```python
from build123d import *

# Parameters (mm, degrees)
BASE_DEPTH          = 3
SERVO_SUPPORT_DEPTH = 43.8
SKETCH21_W          = 6
SKETCH21_H          = 4.65
SERVO_MOUNTS_DEPTH  = 12.4
SERVO_SCREWS_REACH  = 142.173
SKETCH22_R          = 1.3
FILLET1_R           = 2
SKETCH23_W          = 16.5
SKETCH23_H          = 31.3
SHAFT_SUPPORT_DEPTH = 3
SKETCH24_W          = 5.5
SKETCH24_H          = 31.3
BOSS_EXTRUDE6_DEPTH = 56.2
FILLET2_R           = 8
FILLET3_R           = 8
SHAFT_REACH         = 151.771
SKETCH25_R          = 1.7
SCREWS_REACH        = 107.316
SKETCH26_R          = 1.6
SKETCH26_R_2        = 1.4
SKETCH31_W          = 7
SKETCH31_H          = 13.5765
BOSS_EXTRUDE8_DEPTH = 5
SKETCH30_R          = 2.5
BOSS_EXTRUDE9_DEPTH = 2.5
CUT_EXTRUDE1_REACH  = 122.29
SKETCH32_R          = 1.15
CHAMFER1_SIZE       = 2.5
CHAMFER2_SIZE       = 4


with BuildPart() as part:
    # Sketch19 → Base (new body)
    with BuildSketch(Plane.XY):
        Polygon((61.5, 19.3), (56.5, 19.3), (34, 29.3), (34, 34.3), (-59.5, 34.3), (-59.5, -43), (61.5, -43), align=None)
    extrude(amount=BASE_DEPTH)

    # Sketch20 → Servo support (add)
    with BuildSketch(Plane.XY):
        Polygon((-53.298152188, -10.85), (-55.448152188, -10.85), (-59.5, -10.85), (-59.5, 21.25), (-55.448152188, 21.25), (-53.298152188, 21.25), (-45.748152188, 21.25), (-45.748152188, 8.609473612), (-45.748152188, -10.85), align=None)
    extrude(amount=SERVO_SUPPORT_DEPTH)

    # Sketch21 → Servo mounts (add)
    with BuildSketch(Plane.XY.offset(43.8)):
        with Locations((-56.5, -8.525)):
            Rectangle(SKETCH21_W, SKETCH21_H)
        with Locations((-56.5, 18.925)):
            Rectangle(SKETCH21_W, SKETCH21_H)
    extrude(amount=SERVO_MOUNTS_DEPTH)

    # Sketch22 → Servo screws (cut, up to next)
    with BuildSketch(Plane.ZY.offset(59.5), mode=Mode.PRIVATE) as servo_screws_sk1:
        with Locations(Location((50, -8.65, 0), (0, 0, 270))):
            Circle(SKETCH22_R)
    servo_screws_tool1 = extrude(servo_screws_sk1.sketch, amount=-SERVO_SCREWS_REACH, mode=Mode.PRIVATE) & part.part
    # Sketch22 → Servo screws (cut, up to next)
    with BuildSketch(Plane.ZY.offset(59.5), mode=Mode.PRIVATE) as servo_screws_sk2:
        with Locations(Location((50, 19.05, 0), (0, 0, 270))):
            Circle(SKETCH22_R)
    servo_screws_tool2 = extrude(servo_screws_sk2.sketch, amount=-SERVO_SCREWS_REACH, mode=Mode.PRIVATE) & part.part
    add(servo_screws_tool1.solids().sort_by_distance((-59.5, -8.65, 50))[0], mode=Mode.SUBTRACT)
    add(servo_screws_tool2.solids().sort_by_distance((-59.5, 19.05, 50))[0], mode=Mode.SUBTRACT)

    # Fillet1
    fillet1_edges = [part.edges().sort_by_distance(p)[0] for p in [
        (-56.5, 21.25, 56.2),
        (-56.5, -10.85, 56.2),
    ]]
    fillet(fillet1_edges, radius=FILLET1_R)

    # Sketch23 → Shaft support (add)
    with BuildSketch(Plane.XY):
        with Locations((69.75, 3.65)):
            Rectangle(SKETCH23_W, SKETCH23_H)
    extrude(amount=SHAFT_SUPPORT_DEPTH)

    # Sketch24 → Boss-Extrude6 (add)
    with BuildSketch(Plane.XY):
        with Locations((75.25, 3.65)):
            Rectangle(SKETCH24_W, SKETCH24_H)
    extrude(amount=BOSS_EXTRUDE6_DEPTH)

    # Fillet2
    fillet2_edges = [part.edges().sort_by_distance(p)[0] for p in [
        (61.5, -12, 1.5),
    ]]
    fillet(fillet2_edges, radius=FILLET2_R)

    # Fillet3
    fillet3_edges = [part.edges().sort_by_distance(p)[0] for p in [
        (75.25, 19.3, 56.2),
        (75.25, -12, 56.2),
    ]]
    fillet(fillet3_edges, radius=FILLET3_R)

    # Sketch25 → Shaft (cut, up to next)
    with BuildSketch(Plane.ZY.offset(-72.5), mode=Mode.PRIVATE) as shaft_sk1:
        with Locations((50, 0)):
            Circle(SKETCH25_R)
    shaft_tool1 = extrude(shaft_sk1.sketch, amount=-SHAFT_REACH, mode=Mode.PRIVATE) & part.part
    add(shaft_tool1.solids().sort_by_distance((72.5, 0, 50))[0], mode=Mode.SUBTRACT)

    # Sketch26 → Screws (cut, up to next)
    with BuildSketch(Plane.XY, mode=Mode.PRIVATE) as screws_sk1:
        with Locations((-57, -40.5)):
            Circle(SKETCH26_R)
    screws_tool1 = extrude(screws_sk1.sketch, amount=SCREWS_REACH, mode=Mode.PRIVATE) & part.part
    # Sketch26 → Screws (cut, up to next)
    with BuildSketch(Plane.XY, mode=Mode.PRIVATE) as screws_sk2:
        with Locations((-10, -40.5)):
            Circle(SKETCH26_R)
    screws_tool2 = extrude(screws_sk2.sketch, amount=SCREWS_REACH, mode=Mode.PRIVATE) & part.part
    # Sketch26 → Screws (cut, up to next)
    with BuildSketch(Plane.XY, mode=Mode.PRIVATE) as screws_sk3:
        with Locations((59, -32)):
            Circle(SKETCH26_R)
    screws_tool3 = extrude(screws_sk3.sketch, amount=SCREWS_REACH, mode=Mode.PRIVATE) & part.part
    # Sketch26 → Screws (cut, up to next)
    with BuildSketch(Plane.XY, mode=Mode.PRIVATE) as screws_sk4:
        with Locations((59, 16.8)):
            Circle(SKETCH26_R)
    screws_tool4 = extrude(screws_sk4.sketch, amount=SCREWS_REACH, mode=Mode.PRIVATE) & part.part
    # Sketch26 → Screws (cut, up to next)
    with BuildSketch(Plane.XY, mode=Mode.PRIVATE) as screws_sk5:
        with Locations((31.5, 31.8)):
            Circle(SKETCH26_R)
    screws_tool5 = extrude(screws_sk5.sketch, amount=SCREWS_REACH, mode=Mode.PRIVATE) & part.part
    # Sketch26 → Screws (cut, up to next)
    with BuildSketch(Plane.XY, mode=Mode.PRIVATE) as screws_sk6:
        with Locations((-32.5, 31.8)):
            Circle(SKETCH26_R)
    screws_tool6 = extrude(screws_sk6.sketch, amount=SCREWS_REACH, mode=Mode.PRIVATE) & part.part
    # Sketch26 → Screws (cut, up to next)
    with BuildSketch(Plane.XY, mode=Mode.PRIVATE) as screws_sk7:
        with Locations((-57, 25.3)):
            Circle(SKETCH26_R)
    screws_tool7 = extrude(screws_sk7.sketch, amount=SCREWS_REACH, mode=Mode.PRIVATE) & part.part
    # Sketch26 → Screws (cut, up to next)
    with BuildSketch(Plane.XY, mode=Mode.PRIVATE) as screws_sk8:
        with Locations((-57, -14.5)):
            Circle(SKETCH26_R_2)
    screws_tool8 = extrude(screws_sk8.sketch, amount=SCREWS_REACH, mode=Mode.PRIVATE) & part.part
    # Sketch26 → Screws (cut, up to next)
    with BuildSketch(Plane.XY, mode=Mode.PRIVATE) as screws_sk9:
        with Locations((45.5, -40.5)):
            Circle(SKETCH26_R_2)
    screws_tool9 = extrude(screws_sk9.sketch, amount=SCREWS_REACH, mode=Mode.PRIVATE) & part.part
    add(screws_tool1.solids().sort_by_distance((-57, -40.5, 0))[0], mode=Mode.SUBTRACT)
    add(screws_tool2.solids().sort_by_distance((-10, -40.5, 0))[0], mode=Mode.SUBTRACT)
    add(screws_tool3.solids().sort_by_distance((59, -32, 0))[0], mode=Mode.SUBTRACT)
    add(screws_tool4.solids().sort_by_distance((59, 16.8, 0))[0], mode=Mode.SUBTRACT)
    add(screws_tool5.solids().sort_by_distance((31.5, 31.8, 0))[0], mode=Mode.SUBTRACT)
    add(screws_tool6.solids().sort_by_distance((-32.5, 31.8, 0))[0], mode=Mode.SUBTRACT)
    add(screws_tool7.solids().sort_by_distance((-57, 25.3, 0))[0], mode=Mode.SUBTRACT)
    add(screws_tool8.solids().sort_by_distance((-57, -14.5, 0))[0], mode=Mode.SUBTRACT)
    add(screws_tool9.solids().sort_by_distance((45.5, -40.5, 0))[0], mode=Mode.SUBTRACT)

    # Sketch31 → Boss-Extrude8 (add)
    with BuildSketch(Plane.XZ.offset(43)):
        with Locations((0, 9.78825)):
            Rectangle(SKETCH31_W, SKETCH31_H)
        with Locations((58, 9.78825)):
            Rectangle(SKETCH31_W, SKETCH31_H)
    extrude(amount=-BOSS_EXTRUDE8_DEPTH)

    # Sketch30 → Boss-Extrude9 (add)
    with BuildSketch(Plane.XZ.offset(43)):
        with Locations(Location((0, 13.0765, 0), (0, 0, 180))):
            Circle(SKETCH30_R)
        with Locations(Location((58, 13.0765, 0), (0, 0, 180))):
            Circle(SKETCH30_R)
    extrude(amount=BOSS_EXTRUDE9_DEPTH)

    # Sketch32 → Cut-Extrude1 (cut, up to next)
    with BuildSketch(Plane(origin=(0, -38, 0), x_dir=(1, 0, 0), z_dir=(0, 1, 0)), mode=Mode.PRIVATE) as cut_extrude1_sk1:
        with Locations(Location((0, -13.0765, 0), (0, 0, 270))):
            Circle(SKETCH32_R)
    cut_extrude1_tool1 = extrude(cut_extrude1_sk1.sketch, amount=-CUT_EXTRUDE1_REACH, mode=Mode.PRIVATE) & part.part
    # Sketch32 → Cut-Extrude1 (cut, up to next)
    with BuildSketch(Plane(origin=(0, -38, 0), x_dir=(1, 0, 0), z_dir=(0, 1, 0)), mode=Mode.PRIVATE) as cut_extrude1_sk2:
        with Locations(Location((58, -13.0765, 0), (0, 0, 270))):
            Circle(SKETCH32_R)
    cut_extrude1_tool2 = extrude(cut_extrude1_sk2.sketch, amount=-CUT_EXTRUDE1_REACH, mode=Mode.PRIVATE) & part.part
    add(cut_extrude1_tool1.solids().sort_by_distance((0, -38, 13.0765))[0], mode=Mode.SUBTRACT)
    add(cut_extrude1_tool2.solids().sort_by_distance((58, -38, 13.0765))[0], mode=Mode.SUBTRACT)

    # Chamfer1
    # the kernel refuses this chamfer: 2.5 mm, written as the material it adds along each edge
    with BuildSketch(Plane(origin=(58, -43, 13.0765), x_dir=(-1, 0, 0), z_dir=(0, 0, 1))) as chamfer1_piece_1_section:
        Polygon((2.5 + CHAMFER1_SIZE, 0), (2.5, CHAMFER1_SIZE), (2.5, 0), align=None)
    chamfer1_piece_1 = revolve(axis=Axis((58, -43, 13.0765), (0, -1, 0)), mode=Mode.PRIVATE)
    chamfer1_piece_1 = split(chamfer1_piece_1, bisect_by=Plane(origin=(61.5, -43.330528144, 9.079752975), z_dir=(-1, 0, 0)), keep=Keep.TOP, mode=Mode.PRIVATE)
    chamfer1_piece_1 = split(chamfer1_piece_1, bisect_by=Plane(origin=(54.5, -43.330528144, 9.079752975), z_dir=(1, 0, 0)), keep=Keep.TOP, mode=Mode.PRIVATE)
    chamfer1_piece_1 = split(chamfer1_piece_1, bisect_by=Plane(origin=(55.692477029, -43.330528144, 16.5765), z_dir=(0, 0, -1)), keep=Keep.TOP, mode=Mode.PRIVATE)
    chamfer1_piece_1 = split(chamfer1_piece_1, bisect_by=Plane(origin=(55.692477029, -45.5, 9.079752975), z_dir=(0, 1, 0)), keep=Keep.TOP, mode=Mode.PRIVATE)
    add(chamfer1_piece_1)
    with BuildSketch(Plane(origin=(0, -43, 13.0765), x_dir=(-1, 0, 0), z_dir=(0, 0, 1))) as chamfer1_piece_2_section:
        Polygon((2.5 + CHAMFER1_SIZE, 0), (2.5, CHAMFER1_SIZE), (2.5, 0), align=None)
    chamfer1_piece_2 = revolve(axis=Axis((0, -43, 13.0765), (0, -1, 0)), mode=Mode.PRIVATE)
    chamfer1_piece_2 = split(chamfer1_piece_2, bisect_by=Plane(origin=(-3.5, -43.330528144, 9.079752976), z_dir=(1, 0, 0)), keep=Keep.TOP, mode=Mode.PRIVATE)
    chamfer1_piece_2 = split(chamfer1_piece_2, bisect_by=Plane(origin=(-2.30752297, -43.330528144, 16.5765), z_dir=(0, 0, -1)), keep=Keep.TOP, mode=Mode.PRIVATE)
    chamfer1_piece_2 = split(chamfer1_piece_2, bisect_by=Plane(origin=(3.5, -43.330528144, 9.079752976), z_dir=(-1, 0, 0)), keep=Keep.TOP, mode=Mode.PRIVATE)
    chamfer1_piece_2 = split(chamfer1_piece_2, bisect_by=Plane(origin=(-2.30752297, -45.5, 9.079752976), z_dir=(0, 1, 0)), keep=Keep.TOP, mode=Mode.PRIVATE)
    add(chamfer1_piece_2)

    # Chamfer2
    chamfer2_edges = [part.edges().sort_by_distance(p)[0] for p in [
        (72.5, 3.65, 3),
    ]]
    chamfer(chamfer2_edges, length=CHAMFER2_SIZE)


solid = part.part
```
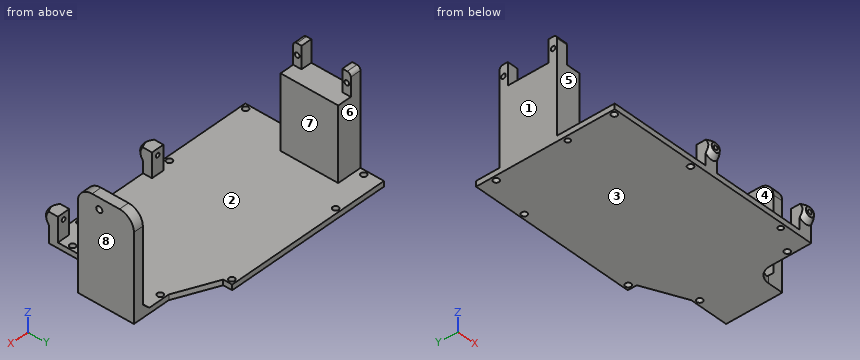
Check sheet for the modelled part. Datum: model origin and axes. Units: mm. Face numbers are marked on the shaded views. A direction names the side the tool comes from. Coordinates: 2 decimals unless noted, no trailing zeros. Loops run counter-clockwise (first coordinate to the right, second up) from the corner with the lowest first, then second, coordinate; pieces in that order, holes last.
1) Sectioned sample at A-A (x = -57). Record the boundary of the cut face in (y, z).
2) Gauge pin test, flat ends, axial feed: pin 1 (3.5 mm diameter, centred on x = 59.5, z = 10, fed in from +Y); pin 2 (4 mm diameter, centred on x = -49, z = 35.5, fed in from +Y); pin 3 (3 mm diameter, centred on x = -57, y = 25.3, fed in from -Z); pin 4 (1.5 mm diameter, centred on x = -40.5, y = 1, fed in from -Z). Record the tip position at first contact, or that the pin passes through.
3) Release check for a two-part mould opening along X. For the marked faces 1, 2, 3 and 4 record: released by +X, released by -X, zero draft, split by the parting line, or undercut.
4) Access from +Z, -Z, +X, -X, +Y, -Y to the whole of each face (thin tool, end or side, straight path). Record for the marked faces 5, 6, 7 and 8.
5) Material ranges on probe 1 along Y at (x, z) = (-57, 0.75); probe 2 along X at (y, z) = (31.8, 1.9); probe 3 along X at (y, z) = (19, 45), recorded low to high.
6) Sectioned sample at D-D (x = -10). Record the boundary of the cut face in (y, z), and give its area (3 significant figures).
7) Sectioned sample at B-B (y = 31.8). Record the boundary of the cut face in (x, z).
8) Sectioned sample at C-C (z = 22). Record the boundary of the cut face in (x, y), and give its area (3 significant figures).
Check sheet entries:
1. outline: (-43, 0) - (-42.1, 0) - (-42.1, 3) - (-43, 3) - close; (-38.9, 0) - (-15.9, 0) - (-15.9, 3) - (-38.9, 3) - close; (-13.1, 0) - (23.7, 0) - (23.7, 3) - (21.25, 3) - (21.25, 54.2) arc R2 ccw to (19.25, 56.2) - (16.6, 56.2) - (16.6, 43.8) - (-6.2, 43.8) - (-6.2, 56.2) - (-8.85, 56.2) arc R2 ccw to (-10.85, 54.2) - (-10.85, 3) - (-13.1, 3) - close; (26.9, 0) - (34.3, 0) - (34.3, 3) - (26.9, 3) - close; hole circle Ø2.6 at (-8.65, 50); hole circle Ø2.6 at (19.05, 50)
2. pin 1: stops at y = -38
2. pin 2: stops at y = 21.25
2. pin 3: passes through
2. pin 4: stops at z = 0
3. face 1: released by -X
3. face 2: undercut
3. face 3: zero draft
3. face 4: undercut
4. face 5: +Z, -X, -Y
4. face 6: +Z, +X, -X, +Y
4. face 7: +Z, +Y, -Y
4. face 8: +Z, -Z, +X, +Y, -Y
5. probe 1: y = -43 to -42.1, -38.9 to -15.9, -13.1 to 23.7, 26.9 to 34.3
5. probe 2: x = -59.5 to -34.1, -30.9 to 29.9, 33.1 to 34
5. probe 3: x = -59.5 to -53.5, 72.5 to 78
6. outline: (-43, 0) - (-42.1, 0) - (-42.1, 3) - (-43, 3) - close; (-38.9, 0) - (34.3, 0) - (34.3, 3) - (-38.9, 3) - close
6. area: 222 mm2
7. outline: (-59.5, 0) - (-34.1, 0) - (-34.1, 3) - (-59.5, 3) - close; (-30.9, 0) - (29.9, 0) - (29.9, 3) - (-30.9, 3) - close; (33.1, 0) - (34, 0) - (34, 3) - (33.1, 3) - close
8. outline: (-59.5, -10.85) - (-45.75, -10.85) - (-45.75, 21.25) - (-59.5, 21.25) - close; (72.5, -12) - (78, -12) - (78, 19.3) - (72.5, 19.3) - close
8. area: 614 mm2
